```python
from build123d import *

# Parameters (mm, degrees)
SKETCH_W                = 45
SKETCH_H                = 15
PAD_DEPTH               = 3.5
POCKET_DEPTH            = 15.001
LINEARPATTERN_COUNT     = 3
LINEARPATTERN_PITCH     = 15
SKETCH002_W             = 4
SKETCH002_H             = 2
PAD001_DEPTH            = 2.5
SKETCH003_W             = 45
SKETCH003_H             = 15
SKETCH003_W_2           = 43
SKETCH003_H_2           = 13
PAD002_DEPTH            = 9.5
SKETCH004_W             = 1
SKETCH004_H             = 1
PAD003_DEPTH            = 2
SKETCH004_MIRRORED_2_W  = 1
SKETCH004_MIRRORED_2_H  = 1
PAD003_MIRRORED_2_DEPTH = 2
SKETCH005_W             = 3
SKETCH005_H             = 1
SKETCH005_W_2           = 4
PAD004_DEPTH            = 1
CHAMFER_SIZE            = 0.5


with BuildPart() as part:
    # Sketch → Pad (new body)
    with BuildSketch(Plane.XY):
        Rectangle(SKETCH_W, SKETCH_H)
    extrude(amount=PAD_DEPTH)

    # Sketch001 (on Face3 of Pad) → Pocket (cut, through all)
    with BuildSketch(Plane.XZ.offset(7.5)):
        with BuildLine():
            Line((-16.5, 0.722949), (-16.5, 0))
            Line((-16.5, 0), (-13.5, 0))
            Line((-13.5, 0), (-13.5, 0.722949))
            ThreePointArc((-13.5, 0.722949), (-12.87226, 1.668412), (-12.785841, 2.8))
            Line((-17.214159, 2.8), (-12.785841, 2.8))
            ThreePointArc((-17.214159, 2.8), (-17.12774, 1.668412), (-16.5, 0.722949))
        make_face()
    pocket = extrude(amount=-POCKET_DEPTH, mode=Mode.SUBTRACT)

    # LinearPattern: Pocket ×3
    with Locations(*[(i * LINEARPATTERN_PITCH, 0, 0) for i in range(1, LINEARPATTERN_COUNT)]):
        add(pocket, mode=Mode.SUBTRACT)

    # Sketch002 (on Face22 of LinearPattern) → Pad001 (join)
    with BuildSketch(Plane.XY.offset(3.5)):
        with Locations((-19.5, 5.5)):
            Rectangle(SKETCH002_W, SKETCH002_H)
        with Locations((-19.5, -5.5)):
            Rectangle(SKETCH002_W, SKETCH002_H)
        with Locations((19.5, 5.5)):
            Rectangle(SKETCH002_W, SKETCH002_H)
        with Locations((19.5, -5.5)):
            Rectangle(SKETCH002_W, SKETCH002_H)
    extrude(amount=PAD001_DEPTH)

    # Sketch003 (on Face22 of Pad001) → Pad002 (join)
    with BuildSketch(Plane.XY.offset(3.5)):
        Rectangle(SKETCH003_W, SKETCH003_H)
        Rectangle(SKETCH003_W_2, SKETCH003_H_2, mode=Mode.SUBTRACT)
    extrude(amount=PAD002_DEPTH)

    # Sketch004 (on Face37 of Pad002) → Pad003 (join)
    with BuildSketch(Plane.XY.offset(6)):
        with Locations((-18, 6)):
            Rectangle(SKETCH004_W, SKETCH004_H)
        with Locations((-21, 5)):
            Rectangle(SKETCH004_W, SKETCH004_H)
    pad003 = extrude(amount=PAD003_DEPTH)

    # Sketch004 Mirrored 2 → Pad003 Mirrored 2 (add)
    with BuildSketch(Plane(origin=(0, 0, 6), x_dir=(-1, 0, 0), z_dir=(0, 0, -1))):
        with Locations((-18, 6)):
            Rectangle(SKETCH004_MIRRORED_2_W, SKETCH004_MIRRORED_2_H)
        with Locations((-21, 5)):
            Rectangle(SKETCH004_MIRRORED_2_W, SKETCH004_MIRRORED_2_H)
    pad003_mirrored_2 = extrude(amount=-PAD003_MIRRORED_2_DEPTH)

    # Mirrored001: Pad003, Pad003 Mirrored 2 across Sketch004 H_Axis
    add(pad003.mirror(Plane(origin=(0, 0, 6), x_dir=(0, 0, 1), z_dir=(0, 1, 0))))
    add(pad003_mirrored_2.mirror(Plane(origin=(0, 0, 6), x_dir=(0, 0, 1), z_dir=(0, 1, 0))))

    # Sketch005 (on Face32 of MultiTransform) → Pad004 (join)
    with BuildSketch(Plane.XZ.offset(-6.5)):
        with Locations((-6.82, 12.5)):
            Rectangle(SKETCH005_W, SKETCH005_H)
        with Locations((7.5, 12.5)):
            Rectangle(SKETCH005_W_2, SKETCH005_H)
    pad004 = extrude(amount=PAD004_DEPTH)

    # Mirrored002: Pad004 across XZ
    add(pad004.mirror(Plane.XZ))

    # Chamfer
    chamfer_edges = [part.edges().sort_by_distance(p)[0] for p in [
        (-6.82, 5.5, 13),
        (7.5, 5.5, 13),
        (7.5, -5.5, 13),
        (-6.82, -5.5, 13),
    ]]
    chamfer(chamfer_edges, length=CHAMFER_SIZE)


solid = part.part
```
Here's how the part is built. I have some questions about the finished solid (model axes, mm). A direction names the side the tool comes from. Round coordinates to 2 decimals unless told otherwise and drop trailing zeros. Order: outer loops, then holes, each group sorted by start corner. A loop starts at its lowest first (then second) coordinate and runs counter-clockwise, first axis right, second up. Notation, with made-up numbers: (84, -38.75) -> (109, -38.75) arc R21 cw to (109, -10.75) -> close; hole circle Ø2 at (86, 77). An arc over 180 degrees is marked (long way). Use a Markdown table: item, result. Add a question column.
(1) Suppose I cut it at D-D, the plane z = 2.25. Please give me the cut outline in (x, y) (3 decimals).
(2) For pin 1 Ø0.5 at (x, y) = (-21, 5) entering from +Z, with a flat end and sliding along its axis, tell me the tip position at first contact or that it passes through.
(3) For faces 1 (the face through (21, 5, 8)), 2 (the face through (12.87, -0.11, 1.68)), which set-ups out of +Z, -Z, +X, -X, +Y, -Y let a thin tool reach every point of the face, with its end or its side?
(4) Suppose I cut it at A-A, the plane z = 8.5. Please give me the cut outline in (x, y).
(5) If we mould it in two halves opening along Y, with no side actions, what happens to faces 3 (the face through (18, -6, 8)), 4 (the face through (-17.13, -0.11, 1.68))? For each: released by +Y, released by -Y, zero draft, split by the parting line, or undercut.
(6) Suppose I cut it at C-C, the plane y = -2.5. Please give me the cut outline in (x, z), and give its area (3 significant figures).
(7) I need wall thicknesses on line 1 along X through (y, z) = (-5.75, 7.5); line 2 along X through (y, z) = (4.75, 11.5); line 3 along Y through (x, z) = (-13, 9.75). Which ranges of each line are inside material? Lowest first, please.
(8) Suppose I cut it at B-B, the plane x = -14. Please give me the cut outline in (y, z), and give its area (3 significant figures).
Verdict:
| question | item | result |
|---|---|---|
| 1 | outline | (-22.5, -7.5) -> (-17.245, -7.5) -> (-17.245, 7.5) -> (-22.5, 7.5) -> close; (-12.755, -7.5) -> (-2.245, -7.5) -> (-2.245, 7.5) -> (-12.755, 7.5) -> close; (2.245, -7.5) -> (12.755, -7.5) -> (12.755, 7.5) -> (2.245, 7.5) -> close; (17.245, -7.5) -> (22.5, -7.5) -> (22.5, 7.5) -> (17.245, 7.5) -> close |
| 2 | pin 1 | z = 8 |
| 3 | face 1 | +Z |
| 3 | face 2 | +Y, -Y |
| 4 | outline | (-22.5, -7.5) -> (22.5, -7.5) -> (22.5, 7.5) -> (-22.5, 7.5) -> close; hole (-21.5, -6.5) -> (21.5, -6.5) -> (21.5, 6.5) -> (-21.5, 6.5) -> close |
| 5 | face 3 | undercut |
| 5 | face 4 | zero draft |
| 6 | outline | (-22.5, 0) -> (-16.5, 0) -> (-16.5, 0.72) arc R2.25 cw to (-17.21, 2.8) -> (-12.79, 2.8) arc R2.25 cw to (-13.5, 0.72) -> (-13.5, 0) -> (-1.5, 0) -> (-1.5, 0.72) arc R2.25 cw to (-2.21, 2.8) -> (2.21, 2.8) arc R2.25 cw to (1.5, 0.72) -> (1.5, 0) -> (13.5, 0) -> (13.5, 0.72) arc R2.25 cw to (12.79, 2.8) -> (17.21, 2.8) arc R2.25 cw to (16.5, 0.72) -> (16.5, 0) -> (22.5, 0) -> (22.5, 13) -> (21.5, 13) -> (21.5, 3.5) -> (-21.5, 3.5) -> (-21.5, 13) -> (-22.5, 13) -> close |
| 6 | area | 144 mm2 |
| 7 | line 1 | -22.5 to -21.5, -18.5 to -17.5, 17.5 to 18.5, 21.5 to 22.5 |
| 7 | line 2 | -22.5 to -21.5, 21.5 to 22.5 |
| 7 | line 3 | -7.5 to -6.5, 6.5 to 7.5 |
| 8 | outline | (-7.5, 2.8) -> (7.5, 2.8) -> (7.5, 13) -> (6.5, 13) -> (6.5, 3.5) -> (-6.5, 3.5) -> (-6.5, 13) -> (-7.5, 13) -> close |
| 8 | area | 29.5 mm2 |
